Input: dimensioned drawing with shaded views. Units: mm. Origin: part minimum x, y, z. A direction names the side the tool comes from. Round coordinates to 2 decimals unless told otherwise and drop trailing zeros. Write each loop counter-clockwise with the first axis right and the second up, starting at its lowest first coordinate (ties: lowest second). Pieces come first, ordered by that corner, then holes. Notation, with made-up numbers: M 29,34.25 L 67,34.25 A26 ccw 67,50.25 Z; hole C -20.5,35.25 d9. An arc over 180 degrees is marked long. Answer in a Markdown table with one row per item. Add a question column.
Item 1: Cut plane B-B on y = 7.5. Return loops of the section in (x, z).
Item 2: Set-up query: the marked faces 1, 2 and 3. Return all of +Z, -Z, +X, -X, +Y, -Y with unobstructed straight access to the full face (end or side cutting, diameter ignored); none if empty.
Item 3: Cut plane A-A on x = 27. Return loops of the section in (y, z).
Item 4: Material intervals for probe 1 along Y at (x, z) = (5.5, 6.75); probe 2 along Z at (x, y) = (16.5, 2.45); probe 3 along X at (y, z) = (17, 5.5), sorted ascending.
Item 5: Cut plane C-C on x = 16.5. Return loops of the section in (y, z).
Item 6: Contact query for flat-ended pins moving along their axis: pin 1 (4 mm diameter, centred on x = 12, z = 10, fed in from +Y); pin 2 (11 mm diameter, centred on x = 16.5, z = 19, fed in from +Y) (3 decimals); pin 3 (1.8 mm diameter, centred on y = 15.5, z = 9.5, fed in from +X). Output: stop coordinate, or through.
Item 7: Mould query, pull axis X, two halves, no side actions, for the marked faces 4 and 5. Classes: released by +X, released by -X, zero draft, split by the parting line, or undercut.
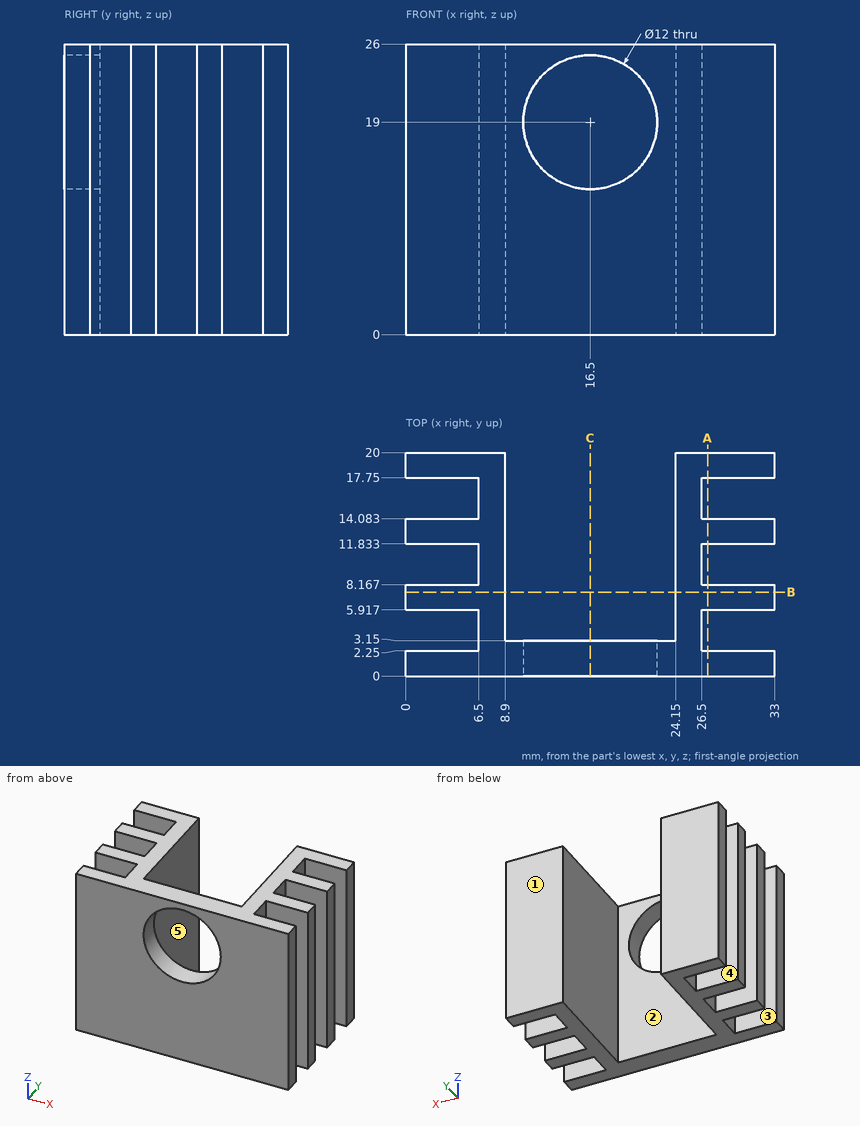
Results below:
| question | item | result |
|---|---|---|
| 1 | outline | M 0,0 L 8.9,0 L 8.9,26 L 0,26 Z; M 24.15,0 L 33,0 L 33,26 L 24.15,26 Z |
| 2 | face 1 | +Z, -Z, +X, -X, +Y |
| 2 | face 2 | +Z, -Z, +Y |
| 2 | face 3 | +Z, -Z, -X |
| 3 | outline | M 0,0 L 2.25,0 L 2.25,26 L 0,26 Z; M 5.92,0 L 8.17,0 L 8.17,26 L 5.92,26 Z; M 11.83,0 L 14.08,0 L 14.08,26 L 11.83,26 Z; M 17.75,0 L 20,0 L 20,26 L 17.75,26 Z |
| 4 | probe 1 | 0 to 2.25, 5.92 to 8.17, 11.83 to 14.08, 17.75 to 20 |
| 4 | probe 2 | 0 to 13, 25 to 26 |
| 4 | probe 3 | 6.5 to 8.9, 24.15 to 26.5 |
| 5 | outline | M 0,0 L 3.15,0 L 3.15,13 L 0,13 Z; M 0,25 L 3.15,25 L 3.15,26 L 0,26 Z |
| 6 | pin 1 | y = 3.15 |
| 6 | pin 2 | through |
| 6 | pin 3 | x = 26.5 |
| 7 | face 4 | zero draft |
| 7 | face 5 | undercut |
